from build123d import *

# Parameters (mm, degrees)
ESQUISSE1_W                    = 5
ESQUISSE1_H                    = 45
BOSS_EXTRU_1_DEPTH             = 5
CARR_DEPTH                     = 10
CARR_DEPTH_BACK                = 129
ESQUISSE7_W                    = 5.65685425
ESQUISSE7_H                    = 5.65685425
BOSS_EXTRU_3_REACH             = 108.655
BOSS_EXTRU_3_DIRECTION_2_REACH = 108.655
R_P_TITION_LIN_AIRE1_COUNT     = 14
R_P_TITION_LIN_AIRE1_PITCH     = 3.141592
ESQUISSE8_R                    = 1
ENL_V_MAT_EXTRU_3_DEPTH        = 10
ENL_V_START                    = -10
ESQUISSE9_R                    = 1
ENL_V_MAT_EXTRU_4_DEPTH        = 10


with BuildPart() as part:
    # Esquisse1 → Boss.-Extru.1 (new body)
    with BuildSketch(Plane(origin=(0, 0, 0), x_dir=(1, 0, 0), z_dir=(0, 1, 0))):
        Rectangle(ESQUISSE1_W, ESQUISSE1_H)
    extrude(amount=BOSS_EXTRU_1_DEPTH)

    # Esquisse7 → Carr (add, two sides: drawn at the far end of the back side and taken through both)
    with BuildSketch(Plane(origin=(0, 0, -22.5), x_dir=(-1, 0, 0), z_dir=(0, 0, -1)).offset(-CARR_DEPTH_BACK)):
        Rectangle(ESQUISSE7_W, ESQUISSE7_H)
    extrude(amount=CARR_DEPTH + CARR_DEPTH_BACK)

    # Boss.-Extru.3: up to this face of the body (flat: up to its plane)
    boss_extru_3_end = Plane(part.part.faces().sort_by_distance((2.5, 3.914213562, 0))[0])
    # Esquisse3 → Boss.-Extru.3 (add, up to the picked face)
    with BuildSketch(Plane(origin=(0, 0, 0), x_dir=(0, 0, -1), z_dir=(1, 0, 0)), mode=Mode.PRIVATE) as boss_extru_3_sk1:
        with BuildLine():
            Line((19.381081141, 5), (21.5, 5))
            Line((21.5, 5), (20.828241228, 7.270751612))
            ThreePointArc((20.828241228, 7.270751612), (20.440540571, 7.273642384), (20.052839914, 7.270751612))
            Line((20.052839914, 7.270751612), (19.381081141, 5))
        make_face()
    boss_extru_3_tool1 = split(extrude(boss_extru_3_sk1.sketch, amount=BOSS_EXTRU_3_REACH, mode=Mode.PRIVATE), bisect_by=boss_extru_3_end, keep=Keep.BOTH, mode=Mode.PRIVATE)
    boss_extru_3 = boss_extru_3_tool1.solids().sort_by(Axis((0, 5.960295, -20.440541), (1, 0, 0)))[0]
    add(boss_extru_3)

    # Boss.-Extru.3 direction 2: up to this face of the body (flat: up to its plane)
    boss_extru_3_direction_2_end = Plane(part.part.faces().sort_by_distance((-2.5, 3.914213562, 0))[0])
    # Esquisse3 → Boss.-Extru.3 direction 2 (add, up to the picked face)
    with BuildSketch(Plane(origin=(0, 0, 0), x_dir=(0, 0, -1), z_dir=(1, 0, 0)), mode=Mode.PRIVATE) as boss_extru_3_direction_2_sk1:
        with BuildLine():
            Line((19.381081141, 5), (21.5, 5))
            Line((21.5, 5), (20.828241228, 7.270751612))
            ThreePointArc((20.828241228, 7.270751612), (20.440540571, 7.273642384), (20.052839914, 7.270751612))
            Line((20.052839914, 7.270751612), (19.381081141, 5))
        make_face()
    boss_extru_3_direction_2_tool1 = split(extrude(boss_extru_3_direction_2_sk1.sketch, amount=-BOSS_EXTRU_3_DIRECTION_2_REACH, mode=Mode.PRIVATE), bisect_by=boss_extru_3_direction_2_end, keep=Keep.BOTH, mode=Mode.PRIVATE)
    boss_extru_3_direction_2 = boss_extru_3_direction_2_tool1.solids().sort_by(Axis((0, 5.960295, -20.440541), (-1, 0, 0)))[0]
    add(boss_extru_3_direction_2)

    # R_p_tition lin_aire1: Boss.-Extru.3, Boss.-Extru.3 direction 2 ×14
    with Locations(*[(0, 0, i * R_P_TITION_LIN_AIRE1_PITCH) for i in range(1, R_P_TITION_LIN_AIRE1_COUNT)]):
        add(boss_extru_3)
        add(boss_extru_3_direction_2)

    # Esquisse8 → Enl_v. mat.-Extru.3 (cut)
    with BuildSketch(Plane(origin=(0, 0, -32.5), x_dir=(-1, 0, 0), z_dir=(0, 0, -1))):
        Circle(ESQUISSE8_R)
    extrude(amount=-ENL_V_MAT_EXTRU_3_DEPTH, mode=Mode.SUBTRACT)

    # Esquisse9 → Enl_v. mat.-Extru.4 (cut)
    with BuildSketch(Plane.XY.offset(106.5).offset(ENL_V_START)):
        with Locations(Location((0, 0, 0), (0, 0, 180))):
            Circle(ESQUISSE9_R)
    extrude(amount=ENL_V_MAT_EXTRU_4_DEPTH, mode=Mode.SUBTRACT)


solid = part.part
Work out the finished part from the listing and answer in its coordinate system (mm). A direction names the side the tool comes from. Coordinates: 2 decimals unless noted, no trailing zeros. Write each loop counter-clockwise with the first axis right and the second up, starting at its lowest first coordinate (ties: lowest second). Pieces come first, ordered by that corner, then holes. Notation, with made-up numbers: M -30,-29.5 L -13,-29.5 A18 cw -13,-21.5 Z; hole C 86,54.5 d2. An arc over 180 degrees is marked long. Answer as CSV lines item,"result". Start each with the question number.
Item 1: Determine the mould class of faces 1 (the face through (-0.035, 6.119, 0.822)), 2 (the face through (-0.04, 6.15, 21.12)), 3 (the face through (0, 4, -22.5)) for opening direction Z: released by +Z, released by -Z, zero draft, split by the parting line, or undercut.
Item 2: Consider L1, parallel to Y at x = 0, z = 101.25; L2, parallel to Y at x = 2.5, z = 50.5; L3, parallel to Y at x = 0.1, z = -18.5. Determine where each line is inside the solid, lowest interval first.
Item 3: A tool of negligible diameter and unlimited length cuts with its end or side. For faces 4 (the face through (2.828, 0, 38)), 5 (the face through (-2.5, 4.5, 0.3)), 6 (the face through (2.5, 4.5, 0.3)), 7 (the face through (0.035, 6.119, -18.027)), 8 (the face through (0, 4, 22.5)), from which of +Z, -Z, +X, -X, +Y, -Y can it reach the whole face along a straight path? Write none if from no direction.
Item 4: Section A-A on z = 39.5 is taken. Write down the section's boundary in (x, y).
Item 5: Flat-ended cylindrical pins translate along their axes: P1, Ø0.5, axis at x = 0, z = -12.5, coming from the +Y side; P2, Ø1.5, axis at x = -1.5, z = 36, coming from the +Y side. Find the tip coordinate at first contact, or state that the pin passes through.
Checks:
1,face 1,"undercut"
1,face 2,"released by +Z"
1,face 3,"released by -Z"
2,L1,"y = -2.83 to -1, 1 to 2.83"
2,L2,"y = -2.83 to 2.83"
2,L3,"y = -2.83 to 5"
3,face 4,"+Z, -Z, +X, +Y, -Y"
3,face 5,"+Z, -Z, -X, +Y"
3,face 6,"+Z, -Z, +X, +Y"
3,face 7,"+X, -X, +Y"
3,face 8,"+Z, +X, -X, +Y"
4,outline,"M -2.83,-2.83 L 2.83,-2.83 L 2.83,2.83 L -2.83,2.83 Z"
5,P1,"stops at y = 5"
5,P2,"stops at y = 2.83"
